The listing builds one solid part. Answer for the finished solid, in the listing's coordinates (mm). A direction names the side the tool comes from. Round coordinates to 2 decimals unless told otherwise and drop trailing zeros. Loops run counter-clockwise (first coordinate to the right, second up) from the corner with the lowest first, then second, coordinate; pieces in that order, holes last. Notation, with made-up numbers: (12.5, 66) - (20.5, 66) arc R31 cw to (20.5, 104) - close; hole circle Ø3 at (-15, 68). An arc over 180 degrees is marked (long way). One line per item, written item: value.
```python
from build123d import *

# Parameters (mm, degrees)
SKETCH1_R           = 3.25
BOSS_EXTRUDE1_DEPTH = 2.46
SKETCH2_R           = 1.75
CUT_EXTRUDE1_DEPTH  = 3.35
SKETCH6_R           = 4.8
BOSS_EXTRUDE2_DEPTH = 5
FILLET1_R           = 0.75


with BuildPart() as part:
    # Sketch1 → Boss-Extrude1 (new body)
    with BuildSketch(Plane(origin=(0, 0, 0), x_dir=(1, 0, 0), z_dir=(0, 1, 0))):
        Circle(SKETCH1_R)
    extrude(amount=BOSS_EXTRUDE1_DEPTH)

    # Sketch2 → Cut-Extrude1 (cut)
    with BuildSketch(Plane.XZ):
        Circle(SKETCH2_R)
    extrude(amount=-CUT_EXTRUDE1_DEPTH, mode=Mode.SUBTRACT)

    # Sketch6 → Boss-Extrude2 (add)
    with BuildSketch(Plane(origin=(0, 2.46, 0), x_dir=(1, 0, 0), z_dir=(0, 1, 0))):
        Circle(SKETCH6_R)
    extrude(amount=BOSS_EXTRUDE2_DEPTH)

    # Fillet1
    fillet1_edges = [part.edges().sort_by_distance(p)[0] for p in [
        (-4.8, 7.46, 0),
    ]]
    fillet(fillet1_edges, radius=FILLET1_R)


solid = part.part
```
1) A cutting plane is placed at B-B on z = 0. Give the vertices of the cut face in (x, y).
Final values:
outline: (-4.8, 2.46) - (-3.25, 2.46) - (-3.25, 0) - (-1.75, 0) - (-1.75, 2.46) - (1.75, 2.46) - (1.75, 0) - (3.25, 0) - (3.25, 2.46) - (4.8, 2.46) - (4.8, 6.71) arc R0.75 ccw to (4.05, 7.46) - (-4.05, 7.46) arc R0.75 ccw to (-4.8, 6.71) - close
2) A cutting plane is placed at C-C on x = 0. Give the vertices of the cut face in (y, z), and give its area (3 significant figures).
Final values:
outline: (0, -3.25) - (2.46, -3.25) - (2.46, -4.8) - (6.71, -4.8) arc R0.75 ccw to (7.46, -4.05) - (7.46, 4.05) arc R0.75 ccw to (6.71, 4.8) - (2.46, 4.8) - (2.46, 3.25) - (0, 3.25) - (0, 1.75) - (2.46, 1.75) - (2.46, -1.75) - (0, -1.75) - close
area: 55.1 mm2
3) For faces 1 (the cylindrical face through (1.617, 1.213, -0.67)), 2 (the flat face through (1.4, 0, 1.4)), determine the directions among +Z, -Z, +X, -X, +Y, -Y from which every point of the face is accessible in a straight line to the end or side of a thin tool.
Final values:
face 1: -Y
face 2: +Z, -Z, +X, -X, -Y
4) For a pull along X with two mould halves and no side action, classify faces 3 (the cylindrical face through (-2.579, 1.213, 1.978)), 4 (the flat face through (0, 2.46, 0)), 5 (the flat face through (0, 7.46, 0)) as released by +X, released by -X, zero draft, split by the parting line, or undercut.
Final values:
face 3: split by the parting line
face 4: undercut
face 5: zero draft
5) A cutting plane is placed at D-D on y = 4. Give the vertices of the cut face in (x, z), and give its area (3 significant figures).
Final values:
outline: circle Ø9.6 at (0, 0)
area: 72.4 mm2
6) Consider L1, parallel to Z at x = 0, y = 1.35; L2, parallel to Y at x = -2.75, z = -3; L3, parallel to X at y = 0.5, z = -0.5. Determine where each line is inside the solid, lowest interval first.
Final values:
L1: -3.25 to -1.75, 1.75 to 3.25
L2: 2.46 to 7.46
L3: -3.21 to -1.68, 1.68 to 3.21
7) A cutting plane is placed at A-A on y = 2. Give the vertices of the cut face in (x, z).
Final values:
outline: circle Ø6.5 at (0, 0); hole circle Ø3.5 at (0, 0)
8) This flat-tipped pin is pushed along its axis until it touches: pin 1 Ø4 at (x, y) = (-3, 2) entering from +Z. Where does it stop, or does it pass through?
Final values:
pin 1: z = 4.68
